```python
from build123d import *

# Parameters (mm, degrees)
SKETCH_1_R      = 1
EXTRUDE_2_DEPTH = 0.5


with BuildPart() as part:
    # Эскиз1 → Бобышка-Вытянуть2 (new body)
    with BuildSketch(Plane.XY):
        with BuildLine():
            Line((-0.75, 6.253845396), (-0.75, 1.984313483))
            ThreePointArc((-0.75, 1.984313483), (-0.780777178, 1.877713125), (-0.863636364, 1.803921348))
            ThreePointArc((-0.863636364, 1.803921348), (-1.732050808, 1), (-1.994059896, -0.154029644))
            ThreePointArc((-1.994059896, -0.154029644), (-2.016535856, -0.262683692), (-2.093465886, -0.342637689))
            Line((-2.093465886, -0.342637689), (-5.790988984, -2.477403645))
            ThreePointArc((-5.790988984, -2.477403645), (-5.952066421, -2.494644217), (-6.073072206, -2.38693731))
            ThreePointArc((-6.073072206, -2.38693731), (-6.750627118, -0.327987365), (-6.968602233, 1.828593814))
            ThreePointArc((-6.968602233, 1.828593814), (-7.099193079, 1.978512308), (-7.263875102, 1.867115022))
            ThreePointArc((-7.263875102, 1.867115022), (-6.495190528, -3.75), (-2.01496851, -7.224257879))
            ThreePointArc((-2.01496851, -7.224257879), (-1.836154619, -7.137337707), (-1.90069242, -6.949283469))
            ThreePointArc((-1.90069242, -6.949283469), (-3.659358949, -5.682220893), (-5.103684451, -4.065966154))
            ThreePointArc((-5.103684451, -4.065966154), (-5.136458476, -3.907318617), (-5.040988984, -3.776441751))
            Line((-5.040988984, -3.776441751), (-1.343465886, -1.641675794))
            ThreePointArc((-1.343465886, -1.641675794), (-1.235758679, -1.615029433), (-1.130423532, -1.649891705))
            ThreePointArc((-1.130423532, -1.649891705), (0, -2), (1.130423532, -1.649891705))
            ThreePointArc((1.130423532, -1.649891705), (1.235758679, -1.615029433), (1.343465886, -1.641675794))
            Line((1.343465886, -1.641675794), (5.040988984, -3.776441751))
            ThreePointArc((5.040988984, -3.776441751), (5.136458476, -3.907318617), (5.103684451, -4.065966154))
            ThreePointArc((5.103684451, -4.065966154), (3.659358949, -5.682220893), (1.90069242, -6.949283469))
            ThreePointArc((1.90069242, -6.949283469), (1.836154619, -7.137337707), (2.01496851, -7.224257879))
            ThreePointArc((2.01496851, -7.224257879), (6.495190528, -3.75), (7.263875102, 1.867115022))
            ThreePointArc((7.263875102, 1.867115022), (7.099193079, 1.978512308), (6.968602233, 1.828593814))
            ThreePointArc((6.968602233, 1.828593814), (6.750627118, -0.327987365), (6.073072206, -2.38693731))
            ThreePointArc((6.073072206, -2.38693731), (5.952066421, -2.494644217), (5.790988984, -2.477403645))
            Line((5.790988984, -2.477403645), (2.093465886, -0.342637689))
            ThreePointArc((2.093465886, -0.342637689), (2.016535856, -0.262683692), (1.994059896, -0.154029644))
            ThreePointArc((1.994059896, -0.154029644), (1.732050808, 1), (0.863636364, 1.803921348))
            ThreePointArc((0.863636364, 1.803921348), (0.780777178, 1.877713125), (0.75, 1.984313483))
            Line((0.75, 1.984313483), (0.75, 6.253845396))
            ThreePointArc((0.75, 6.253845396), (0.815607945, 6.401962834), (0.969387755, 6.452903465))
            ThreePointArc((0.969387755, 6.452903465), (3.091268168, 6.010208258), (5.067909813, 5.120689655))
            ThreePointArc((5.067909813, 5.120689655), (5.26303846, 5.158825399), (5.248906592, 5.357142857))
            ThreePointArc((5.248906592, 5.357142857), (0, 7.5), (-5.248906592, 5.357142857))
            ThreePointArc((-5.248906592, 5.357142857), (-5.26303846, 5.158825399), (-5.067909813, 5.120689655))
            ThreePointArc((-5.067909813, 5.120689655), (-3.091268168, 6.010208258), (-0.969387755, 6.452903465))
            ThreePointArc((-0.969387755, 6.452903465), (-0.815607945, 6.401962834), (-0.75, 6.253845396))
        make_face()
        Circle(SKETCH_1_R, mode=Mode.SUBTRACT)
    extrude(amount=EXTRUDE_2_DEPTH)


solid = part.part
```
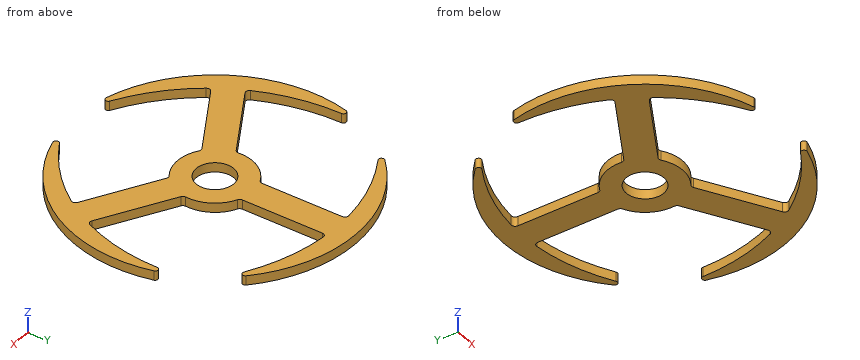
Model file for the job. Use its own axes, mm. Coordinates: 2 decimals unless noted, no trailing zeros. Order: outer loops, then holes, each group sorted by start corner. A loop starts at its lowest first (then second) coordinate and runs counter-clockwise, first axis right, second up. Notation, with made-up numbers: (12, -13) -> (17, -13) arc R27 cw to (17, 8) -> close; hole circle Ø4 at (43.5, -12.5). An arc over 180 degrees is marked (long way). Answer as a JSON object with one key per item and string values. Group by question number.
1) Cut at A-A, the plane x = 0. Write the cut outline in (y, z).
2) Flat gauge pin, fed straight in: pin 1 (1.6 mm diameter, centred on x = 0, y = 0, fed in from -Z). Where does the tip first touch, or does it go through?
3) Cut at C-C, the plane x = 4. Write the cut outline in (y, z).
4) Cut at D-D, the plane x = -6.25. Write the cut outline in (y, z).
5) Drill centre lines: L1, parallel to Y at x = -4, z = 0.15; L2, parallel to X at y = -0.25, z = 0.15; L3, parallel to X at y = -0.5, z = 0.35. Where is each one in solid material? Low to high.
6) Cut at B-B, the plane x = -4.5. Write the cut outline in (y, z), then the cut area to 3 significant figures.
Check values:
{
 "1": {"outline": "(-2, 0) -> (-1, 0) -> (-1, 0.5) -> (-2, 0.5) -> close; (1, 0) -> (7.5, 0) -> (7.5, 0.5) -> (1, 0.5) -> close"},
 "2": {"pin 1": "passes through"},
 "3": {"outline": "(-6.34, 0) -> (-5.36, 0) -> (-5.36, 0.5) -> (-6.34, 0.5) -> close; (-3.18, 0) -> (-1.44, 0) -> (-1.44, 0.5) -> (-3.18, 0.5) -> close; (5.67, 0) -> (6.34, 0) -> (6.34, 0.5) -> (5.67, 0.5) -> close"},
 "4": {"outline": "(-4.15, 0) -> (-1.97, 0) -> (-1.97, 0.5) -> (-4.15, 0.5) -> close"},
 "5": {"L1": "y = -6.34 to -5.36, -3.18 to -1.44, 5.67 to 6.34", "L2": "x = -7.5 to -6.77, -2.01 to -0.97, 0.97 to 2.01, 6.77 to 7.5", "L3": "x = -7.48 to -6.71, -2.37 to -0.87, 0.87 to 2.37, 6.71 to 7.48"},
 "6": {"outline": "(-6, 0) -> (-4.83, 0) -> (-4.83, 0.5) -> (-6, 0.5) -> close; (-3.46, 0) -> (-1.73, 0) -> (-1.73, 0.5) -> (-3.46, 0.5) -> close; (5.43, 0) -> (6, 0) -> (6, 0.5) -> (5.43, 0.5) -> close", "area": "1.74 mm²"}
}
